The listing builds one solid part. Answer for the finished solid, in the listing's coordinates (mm). Round coordinates to 2 decimals unless told otherwise and drop trailing zeros. Order: outer loops, then holes, each group sorted by start corner. A loop starts at its lowest first (then second) coordinate and runs counter-clockwise, first axis right, second up. Notation, with made-up numbers: (-32, 36.5) - (-27, 36.5) arc R20 ccw to (-27, 59.5) - close; hole circle Ø8 at (4.5, 44). An arc over 180 degrees is marked (long way). Use CSV: the item, a comma, the result in double quotes. Start each with the question number.
Item 1: Find section C-C, the plane z = 0.6. Count the separate pieces of the cut face and the enclosed holes in it, plus the area to 3 significant figures.
Item 2: Straight lines are drawn through the part: line 1 along Y through (x, z) = (-19.5, 2.9); line 2 along X through (y, z) = (-4, 3.5); line 3 along Y through (x, z) = (-35, 1.7). For each, find the intervals that lie inside material, in ascending order. Write a range as [from, to].
Item 3: A flat-ended cylindrical pin translates along its axis: P1, Ø4.5, axis at x = -15.97, y = 0, coming from the +Z side. Find the tip coordinate at first contact, or state that the pin passes through.
Item 4: Find section B-B, the plane x = -35. Give the vertices of the cut face in (y, z).
Item 5: Find section A-A, the plane y = 35. Give the vertices of the cut face in (x, z).
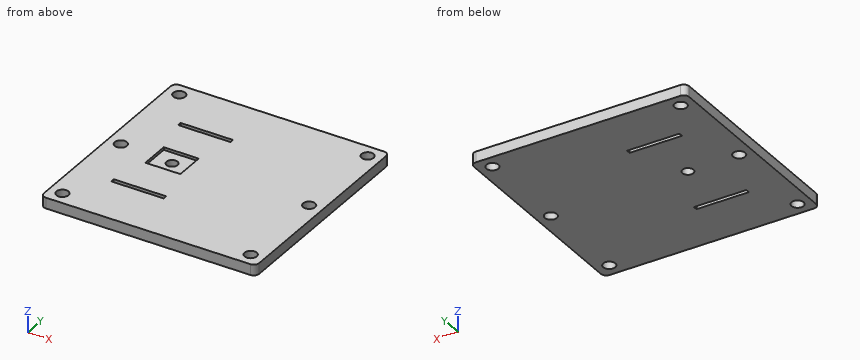
```python
from build123d import *

# Parameters (mm, degrees)
F0_R     = 2.25
F1_DEPTH = 4
F2_R     = 2.05
F3_DEPTH = 5
F4_W     = 13
F4_H     = 11
F5_DEPTH = 1
F6_W     = 19.5
F6_H     = 1.5
F7_DEPTH = 25


# Not quite as in the source:
# - a feature names something its author has since deleted; it is built from what else it names


with BuildPart() as f1:
    # F0 (on Top) → F1 (new body)
    with BuildSketch(Plane.XY):
        with BuildLine():
            ThreePointArc((40, 38), (39.4142135624, 39.4142135624), (38, 40))
            Line((38, 40), (-38, 40))
            ThreePointArc((-38, 40), (-39.4142135624, 39.4142135624), (-40, 38))
            Line((-40, 38), (-40, -38))
            ThreePointArc((-40, -38), (-39.4142135624, -39.4142135624), (-38, -40))
            Line((-38, -40), (38, -40))
            ThreePointArc((38, -40), (39.4142135624, -39.4142135624), (40, -38))
            Line((40, -38), (40, 38))
        make_face()
        with Locations((-35, -35)):
            Circle(F0_R, mode=Mode.SUBTRACT)
        with Locations((35, -35)):
            Circle(F0_R, mode=Mode.SUBTRACT)
        with Locations((-35, 0)):
            Circle(F0_R, mode=Mode.SUBTRACT)
        with Locations((-35, 35)):
            Circle(F0_R, mode=Mode.SUBTRACT)
        with Locations((35, 0)):
            Circle(F0_R, mode=Mode.SUBTRACT)
        with Locations((35, 35)):
            Circle(F0_R, mode=Mode.SUBTRACT)
    extrude(amount=F1_DEPTH)

    # F2 (on face) → F3 (cut)
    with BuildSketch(Plane.XY.offset(4)):
        with Locations((-15.9661, 0)):
            Circle(F2_R)
    extrude(amount=-F3_DEPTH, mode=Mode.SUBTRACT)

    # F4 (on face) → F5 (cut)
    with BuildSketch(Plane.XY.offset(4)):
        with Locations((-15.9661, 0)):
            Rectangle(F4_W, F4_H)
    extrude(amount=-F5_DEPTH, mode=Mode.SUBTRACT)

    # F6 (on face) → F7 (cut)
    with BuildSketch(Plane.XY.offset(4)):
        with Locations((-15.9661, 20)):
            Rectangle(F6_W, F6_H)
        with Locations((-15.9661, -20)):
            Rectangle(F6_W, F6_H)
    extrude(amount=-F7_DEPTH, mode=Mode.SUBTRACT)


solid = f1.part
```
Worked out:
1,separate pieces,"1"
1,enclosed holes,"9"
1,area,"6,230 mm²"
2,line 1,"y = [-40, -20.75], [-19.25, 19.25], [20.75, 40]"
2,line 2,"x = [-40, -22.47], [-9.47, 40]"
2,line 3,"y = [-40, -37.25], [-32.75, -2.25], [2.25, 32.75], [37.25, 40]"
3,P1,"stops at z = 3"
4,outline,"(-40, 0) - (-37.25, 0) - (-37.25, 4) - (-40, 4) - close; (-32.75, 0) - (-2.25, 0) - (-2.25, 4) - (-32.75, 4) - close; (2.25, 0) - (32.75, 0) - (32.75, 4) - (2.25, 4) - close; (37.25, 0) - (40, 0) - (40, 4) - (37.25, 4) - close"
5,outline,"(-40, 0) - (-37.25, 0) - (-37.25, 4) - (-40, 4) - close; (-32.75, 0) - (32.75, 0) - (32.75, 4) - (-32.75, 4) - close; (37.25, 0) - (40, 0) - (40, 4) - (37.25, 4) - close"
